CAD build for the part. Positions are in the model's coordinates, mm. A direction names the side the tool comes from. Coordinates: 2 decimals unless noted, no trailing zeros. Order: outer loops, then holes, each group sorted by start corner. A loop starts at its lowest first (then second) coordinate and runs counter-clockwise, first axis right, second up. Notation, with made-up numbers: M 19.5,38 L 50.5,38 A11 cw 50.5,55 Z; hole C 65.5,30.5 d1. An arc over 180 degrees is marked long. Write item = value, one per line. Start each with the question number.
```python
from build123d import *

# Parameters (mm, degrees)
CROQUIS1_R              = 11
CROQUIS1_R_2            = 3.5
CROQUIS1_R_3            = 1.75
SALIENTE_EXTRUIR1_DEPTH = 3.5
CROQUIS2_R              = 4.9
CROQUIS2_R_2            = 3.5
SALIENTE_EXTRUIR2_DEPTH = 10


with BuildPart() as part:
    # Croquis1 → Saliente-Extruir1 (new body)
    with BuildSketch(Plane(origin=(0, 0, 0), x_dir=(1, 0, 0), z_dir=(0, 1, 0))):
        with Locations(Location((0, 0, 0), (0, 0, 270))):
            Circle(CROQUIS1_R)
        with Locations(Location((0, 0, 0), (0, 0, 270))):
            Circle(CROQUIS1_R_2, mode=Mode.SUBTRACT)
        with Locations(Location((8.25, 0, 0), (0, 0, 270))):
            Circle(CROQUIS1_R_3, mode=Mode.SUBTRACT)
        with Locations(Location((0, 8.25, 0), (0, 0, 270))):
            Circle(CROQUIS1_R_3, mode=Mode.SUBTRACT)
        with Locations(Location((-8.25, 0, 0), (0, 0, 270))):
            Circle(CROQUIS1_R_3, mode=Mode.SUBTRACT)
        with Locations(Location((0, -8.25, 0), (0, 0, 270))):
            Circle(CROQUIS1_R_3, mode=Mode.SUBTRACT)
    extrude(amount=SALIENTE_EXTRUIR1_DEPTH)

    # Croquis2 → Saliente-Extruir2 (add)
    with BuildSketch(Plane(origin=(0, 3.5, 0), x_dir=(1, 0, 0), z_dir=(0, 1, 0))):
        with Locations(Location((0, 0, 0), (0, 0, 270))):
            Circle(CROQUIS2_R)
        with Locations(Location((0, 0, 0), (0, 0, 270))):
            Circle(CROQUIS2_R_2, mode=Mode.SUBTRACT)
    extrude(amount=SALIENTE_EXTRUIR2_DEPTH)


solid = part.part
```
1. Mould opens along Z. For faces 1 (the cylindrical face through (0.526, 1.726, 9.919)), 2 (the cylindrical face through (-10.74, 1.73, -2.38)), 3 (the cylindrical face through (-0.67, 1.726, -6.633)), 4 (the flat face through (3, 0, -3)) say: released by +Z, released by -Z, zero draft, split by the parting line, or undercut.
2. Slice it at B-B (z = 0). Write the cut outline in (x, y), plus the area to 3 significant figures.
3. 3-axis set-ups, long thin cutter, end or side, ignore diameter. For faces 5 (the cylindrical face through (-3.417, 6.656, -0.759)), 6 (the flat face through (-2, 3.5, 5)): which of +Z, -Z, +X, -X, +Y, -Y reach the whole face in a straight line?
4. Slice it at C-C (z = 2.5). Write the cut outline in (x, y), plus the area to 3 significant figures.
5. Flat gauge pins, fed straight in: pin 1 (5.5 mm diameter, centred on x = -8.25, z = 0, fed in from -Y); pin 2 (1.5 mm diameter, centred on x = -7, z = -2.5, fed in from +Y); pin 3 (5 mm diameter, centred on x = -3.5, y = 11, fed in from -Z); pin 4 (3 mm diameter, centred on x = 7, y = 4.5, fed in from -Z). Where does each tip first touch, or does it go through?
6. Probe L1, parallel to X at y = 1.7, z = 0; L2, parallel to X at y = 1.3, z = 8.25; L3, parallel to Y at x = 5.75, z = -5. List the from-to ranges inside material, lowest first.
7. Slice it at D-D (x = -8.25). Write the cut outline in (y, z), plus the area to 3 significant figures.
8. Slice it at A-A (x = 0). Write the cut outline in (y, z), plus the area to 3 significant figures.
Calculated:
q1.face_1 = undercut
q1.face_2 = split by the parting line
q1.face_3 = undercut
q1.face_4 = zero draft
q2.outline = M -11,0 L -10,0 L -10,3.5 L -11,3.5 Z; M -6.5,0 L -3.5,0 L -3.5,13.5 L -4.9,13.5 L -4.9,3.5 L -6.5,3.5 Z; M 3.5,0 L 6.5,0 L 6.5,3.5 L 4.9,3.5 L 4.9,13.5 L 3.5,13.5 Z; M 10,0 L 11,0 L 11,3.5 L 10,3.5 Z
q2.area = 56.0 mm²
q3.face_5 = +Y, -Y
q3.face_6 = +Y
q4.outline = M -10.71,0 L -2.45,0 L -2.45,13.5 L -4.21,13.5 L -4.21,3.5 L -10.71,3.5 Z; M 2.45,0 L 10.71,0 L 10.71,3.5 L 4.21,3.5 L 4.21,13.5 L 2.45,13.5 Z
q4.area = 93.1 mm²
q5.pin_1 = 0
q5.pin_2 = 3.5
q5.pin_3 = -4.8
q5.pin_4 = -9.3
q6.L1 = -11 to -10, -6.5 to -3.5, 3.5 to 6.5, 10 to 11
q6.L2 = -7.28 to -1.75, 1.75 to 7.28
q6.L3 = 0 to 3.5
q7.outline = M 0,-7.28 L 3.5,-7.28 L 3.5,-1.75 L 0,-1.75 Z; M 0,1.75 L 3.5,1.75 L 3.5,7.28 L 0,7.28 Z
q7.area = 38.7 mm²
q8.outline = M 0,-11 L 3.5,-11 L 3.5,-10 L 0,-10 Z; M 0,-6.5 L 3.5,-6.5 L 3.5,-4.9 L 13.5,-4.9 L 13.5,-3.5 L 0,-3.5 Z; M 0,3.5 L 13.5,3.5 L 13.5,4.9 L 3.5,4.9 L 3.5,6.5 L 0,6.5 Z; M 0,10 L 3.5,10 L 3.5,11 L 0,11 Z
q8.area = 56.0 mm²
